from build123d import *

# Parameters (mm, degrees)
CUT_EXTRUDE1_DEPTH      = 199.242276016
CUT_EXTRUDE1_DEPTH_BACK = 199.242276016
SKETCH4_OUTSIDE_W       = 126.226
SKETCH4_OUTSIDE_H       = 126.226
CUT_EXTRUDE2_DEPTH      = 26


with BuildPart() as part:
    # Sketch1 → Revolve1 (revolve)
    with BuildSketch(Plane.XY, mode=Mode.PRIVATE) as revolve1_sk:
        with BuildLine():
            ThreePointArc((27.345454545, 96), (25.880988451, 99.535533906), (22.345454545, 101))
            Line((22.345454545, 101), (20, 101))
            Line((20, 101), (20, 157))
            Line((20, 157), (0, 157))
            Line((0, 157), (0, 190))
            Line((0, 190), (16, 190))
            Line((16, 190), (16, 164))
            Line((16, 164), (30, 164))
            Line((30, 164), (30, 114))
            Line((30, 114), (40, 110))
            Line((40, 110), (27, 0))
            Line((27, 0), (16, 0))
            Line((16, 0), (27.345454545, 96))
        make_face()
    revolve(revolve1_sk.sketch.rotate(Axis((0, 293.194202694, 0), (0, -1, 0)), 90), axis=Axis((0, 293.194202694, 0), (0, -1, 0)))

    # Sketch3 → Cut-Extrude1 (cut, two sides: drawn at the far end of the back side and taken through both)
    with BuildSketch(Plane.XY.offset(-CUT_EXTRUDE1_DEPTH_BACK)):
        Polygon((16, 84), (-16, 84), (-10, 22), (10, 22), align=None)
    extrude(amount=CUT_EXTRUDE1_DEPTH + CUT_EXTRUDE1_DEPTH_BACK, mode=Mode.SUBTRACT)

    # Sketch4 outside → Cut-Extrude2 (cut)
    with BuildSketch(Plane(origin=(0, 190, 0), x_dir=(1, 0, 0), z_dir=(0, 1, 0))):
        Rectangle(SKETCH4_OUTSIDE_W, SKETCH4_OUTSIDE_H)
        Polygon((3.798989873, 16), (16, 3.798989873), (16, -3.798989873), (3.798989873, -16), (-3.798989873, -16), (-16, -3.798989873), (-16, 3.798989873), (-3.798989873, 16), align=None, mode=Mode.SUBTRACT)
    extrude(amount=-CUT_EXTRUDE2_DEPTH, mode=Mode.SUBTRACT)


solid = part.part
Part model, mm, in its own coordinate system. A direction names the side the tool comes from. Coordinates: 2 decimals unless noted, no trailing zeros. Order: outer loops, then holes, each group sorted by start corner. A loop starts at its lowest first (then second) coordinate and runs counter-clockwise, first axis right, second up. Notation, with made-up numbers: M 80.5,89 L 131.5,89 A17 ccw 131.5,107 Z; hole C -36,56 d9. An arc over 180 degrees is marked long. Use a Markdown table: item, result.
(1) Cut at C-C on y = 127. Write the cut outline in (x, z), then the cut area to 3 significant figures.
A:
| item | result |
|---|---|
| outline | C 0,0 d60; hole C 0,0 d40 |
| area | 1,570 mm^2 |
(2) Cut at A-A on x = 0. State how many separate pieces and enclosed holes the cut face has, then the cut area to 3 significant figures.
A:
| item | result |
|---|---|
| separate pieces | 3 |
| enclosed holes | 0 |
| area | 3,450 mm^2 |
(3) Probe L1, parallel to X at y = 131, z = 0; L2, parallel to Y at x = -1, z = 0.5; L3, parallel to Y at x = -1, z = -21.5. List the from-to ranges inside material, lowest first.
A:
| item | result |
|---|---|
| L1 | x = -30 to -20, 20 to 30 |
| L2 | y = 157 to 190 |
| L3 | y = 0 to 22, 101 to 164 |
(4) Flat gauge pins, fed straight in: pin 1 (2 mm diameter, centred on y = 60.5, z = -30, fed in from +X); pin 2 (1 mm diameter, centred on y = 146.5, z = -13, fed in from +X); pin 3 (5 mm diameter, centred on y = 21, z = 26.5, fed in from -X). Where does each tip first touch, or does it go through?
A:
| item | result |
|---|---|
| pin 1 | stops at x = 18.05 |
| pin 2 | stops at x = 27.27 |
| pin 3 | stops at x = -17.16 |
(5) Pull direction Y, two halves, no side cores. Call faces 1 (the flat face through (-13, 53, -25)), 2 (the cylindrical face through (0, 177, -16)), 3 (the conical face through (-9.2, 113.75, 29.21)): released by +Y, released by -Y, zero draft, split by the parting line, or undercut.
A:
| item | result |
|---|---|
| face 1 | undercut |
| face 2 | zero draft |
| face 3 | released by +Y |
(6) Tool access for faces 4 (the flat face through (-14, 164, 7)), 5 (the flat face through (0, 22, -23)), 6 (the cylindrical face through (16, 177, 0)), 7 (the flat face through (-10, 177.2, -9.8)), 8 (the flat face through (-9.8, 177.2, 10)): list every direction of +Z, -Z, +X, -X, +Y, -Y with a clear straight run to the whole face (end or side of a thin tool).
A:
| item | result |
|---|---|
| face 4 | +Y |
| face 5 | +Z, -Z |
| face 6 | +X, +Y |
| face 7 | -Z, -X, +Y |
| face 8 | +Z, -X, +Y |
(7) Cut at B-B on z = 0. Write the cut outline in (x, y), then the cut area to 3 significant figures.
A:
| item | result |
|---|---|
| outline | M -40,110 L -27,0 L -16,0 L -27.35,96 A5 cw -22.35,101 L -20,101 L -20,157 L 20,157 L 20,101 L 22.35,101 A5 cw 27.35,96 L 16,0 L 27,0 L 40,110 L 30,114 L 30,164 L 16,164 L 16,190 L -16,190 L -16,164 L -30,164 L -30,114 Z |
| area | 4,820 mm^2 |
